from build123d import *

# Parameters (mm, degrees)
SKETCH1_W           = 154
SKETCH1_H           = 104
BOSS_EXTRUDE1_DEPTH = 3
FILLET1_R           = 1
SKETCH2_W           = 149
SKETCH2_H           = 99
SKETCH2_W_2         = 145
SKETCH2_H_2         = 95
EXTRUDE_THIN1_DEPTH = 5
FILLET2_R           = 3
FILLET3_R           = 1
CUT_REVOLVE1_ANGLE  = 90
SKETCH5_W           = 50
SKETCH5_H           = 15
CUT_EXTRUDE1_DEPTH  = 1
FILLET4_R           = 0.5
SKETCH6_R           = 2
CUT_EXTRUDE2_DEPTH  = 5
FILLET5_R           = 0.5


with BuildPart() as part:
    # Sketch1 → Boss-Extrude1 (new body)
    with BuildSketch(Plane(origin=(0, 0, 0), x_dir=(1, 0, 0), z_dir=(0, 1, 0))):
        Rectangle(SKETCH1_W, SKETCH1_H)
    extrude(amount=BOSS_EXTRUDE1_DEPTH)

    # Fillet1
    fillet1_edges = [part.edges().sort_by_distance(p)[0] for p in [
        (-77, 3, 0),
        (0, 3, 52),
        (77, 3, 0),
        (77, 1.5, 52),
        (-77, 1.5, 52),
        (-77, 1.5, -52),
        (77, 1.5, -52),
        (0, 3, -52),
    ]]
    fillet(fillet1_edges, radius=FILLET1_R)

    # Sketch2 → Extrude-Thin1 (add)
    with BuildSketch(Plane.XZ):
        Rectangle(SKETCH2_W, SKETCH2_H)
        Rectangle(SKETCH2_W_2, SKETCH2_H_2, mode=Mode.SUBTRACT)
    extrude(amount=EXTRUDE_THIN1_DEPTH)

    # Fillet2
    fillet2_edges = [part.edges().sort_by_distance(p)[0] for p in [
        (72.5, 0, 0),
        (0, 0, 47.5),
        (-72.5, 0, 0),
        (0, 0, -47.5),
    ]]
    fillet(fillet2_edges, radius=FILLET2_R)

    # Fillet3
    fillet3_edges = [part.edges().sort_by_distance(p)[0] for p in [
        (72.5, -5, 0),
        (0, -5, 47.5),
        (-72.5, -5, 0),
        (0, -5, -47.5),
    ]]
    fillet(fillet3_edges, radius=FILLET3_R)

    # Sketch3 → Cut-Revolve1 (revolve, cut)
    with BuildSketch(Plane.ZY.offset(77)):
        with BuildLine():
            Line((-6.5, 0), (6.5, 0))
            ThreePointArc((6.5, 0), (6.060660172, 1.060660172), (5, 1.5))
            Line((5, 1.5), (-5, 1.5))
            ThreePointArc((-5, 1.5), (-6.060660172, 1.060660172), (-6.5, 0))
        make_face()
    revolve(axis=Axis((-77, 0, -6.5), (0, 0, -1)), revolution_arc=CUT_REVOLVE1_ANGLE, mode=Mode.SUBTRACT)

    # Sketch5 → Cut-Extrude1 (cut)
    with BuildSketch(Plane(origin=(0, 3, 0), x_dir=(1, 0, 0), z_dir=(0, 1, 0))):
        with Locations((0, 33.5)):
            Rectangle(SKETCH5_W, SKETCH5_H)
    extrude(amount=-CUT_EXTRUDE1_DEPTH, mode=Mode.SUBTRACT)

    # Fillet4
    fillet4_edges = [part.edges().sort_by_distance(p)[0] for p in [
        (74.5, -2.5, -49.5),
        (74.5, -2.5, 49.5),
        (-74.5, -2.5, 49.5),
        (-74.5, -2.5, -49.5),
    ]]
    fillet(fillet4_edges, radius=FILLET4_R)

    # Sketch6 → Cut-Extrude2 (cut)
    with BuildSketch(Plane(origin=(0, 2, 0), x_dir=(1, 0, 0), z_dir=(0, 1, 0))):
        with Locations(Location((22, 33.5, 0), (0, 0, 270))):
            Circle(SKETCH6_R)
    extrude(amount=-CUT_EXTRUDE2_DEPTH, mode=Mode.SUBTRACT)

    # Fillet5
    fillet5_edges = [part.edges().sort_by_distance(p)[0] for p in [
        (25, 2, -33.5),
        (0, 2, -26),
        (-25, 2, -33.5),
        (0, 2, -41),
    ]]
    fillet(fillet5_edges, radius=FILLET5_R)


solid = part.part
Here's how the part is built. I have some questions about the finished solid (model axes, mm). A direction names the side the tool comes from. Coordinates: 2 decimals unless noted, no trailing zeros. Order: outer loops, then holes, each group sorted by start corner. A loop starts at its lowest first (then second) coordinate and runs counter-clockwise, first axis right, second up. Notation, with made-up numbers: (-5, 55.25) - (0, 55.25) arc R20 ccw to (0, 82.25) - close; hole circle Ø9 at (60, 38). An arc over 180 degrees is marked (long way). Use CSV: the item, a comma, the result in double quotes. Start each with the question number.
1. For faces 1 (the face through (-1, -2, 49.5)), 2 (the face through (-71.64, -0.9, 0.66)), 3 (the face through (21.234, 1.014, -31.653)), which set-ups out of +Z, -Z, +X, -X, +Y, -Y let a thin tool reach every point of the face, with its end or its side?
2. Please list where these lines run through material, in increasing order: line 1 (X direction, y = 1.45, z = -33.5); line 2 (Z direction, x = 40, y = -4.25); line 3 (Y direction, x = 57, z = 3.5). Write a range as from..to.
3. I'm going to push flat-ended pins straight in: pin 1 (6.5 mm diameter, centred on x = 22, z = -33.5, fed in from -Y); pin 2 (0.5 mm diameter, centred on x = -6.5, y = -3.5, fed in from -Z); pin 3 (1 mm diameter, centred on x = 43, y = -4, fed in from +Z). Where does each tip first touch, or does it pass through?
4. Suppose I cut it at B-B on x = 22. List the corners of the cut face in (y, z) for me.
5. Suppose I cut it at C-C on x = -14. List the corners of the cut face in (y, z) for me.
6. If we mould it in two halves opening along X, with no side actions, what happens to faces 4 (the face through (-1, -2, -49.5)), 5 (the face through (74.5, -2, -1)), 6 (the face through (-74.5, -2, -1)), 7 (the face through (0, 2, -34))? For each: +X half, -X half, draft (parallel to the pull), parting line (faces both ways), or undercut.
7. Suppose I cut it at D-D on z = 35. List the corners of the cut face in (x, y) for me, then the cut area to 3 significant figures.
8. Suppose I cut it at A-A on z = -33.5. List the corners of the cut face in (x, y) for me.
Output:
1,face 1,"+Z, +X, -X, -Y"
1,face 2,"-Y"
1,face 3,"+Y, -Y"
2,line 1,"x = -77..20, 24..77"
2,line 2,"z = -49.5..-47.53, 47.53..49.5"
2,line 3,"y = 0..3"
3,pin 1,"stops at y = 0"
3,pin 2,"stops at z = -49.5"
3,pin 3,"stops at z = 49.5"
4,outline,"(-5, -49.5) - (0, -49.5) - (0, -52) - (2, -52) arc R1 ccw to (3, -51) - (3, -41) - (2.5, -41) arc R0.5 cw to (2, -40.5) - (2, -35.5) - (0, -35.5) - (0, -44.5) arc R3 cw to (-3, -47.5) - (-4, -47.5) arc R1 ccw to (-5, -48.5) - close; (-5, 48.5) arc R1 ccw to (-4, 47.5) - (-3, 47.5) arc R3 cw to (0, 44.5) - (0, -31.5) - (2, -31.5) - (2, -26.5) arc R0.5 cw to (2.5, -26) - (3, -26) - (3, 51) arc R1 ccw to (2, 52) - (0, 52) - (0, 49.5) - (-5, 49.5) - close"
5,outline,"(-5, -49.5) - (0, -49.5) - (0, -52) - (2, -52) arc R1 ccw to (3, -51) - (3, -41) - (2.5, -41) arc R0.5 cw to (2, -40.5) - (2, -26.5) arc R0.5 cw to (2.5, -26) - (3, -26) - (3, 51) arc R1 ccw to (2, 52) - (0, 52) - (0, 49.5) - (-5, 49.5) - (-5, 48.5) arc R1 ccw to (-4, 47.5) - (-3, 47.5) arc R3 cw to (0, 44.5) - (0, -44.5) arc R3 cw to (-3, -47.5) - (-4, -47.5) arc R1 ccw to (-5, -48.5) - close"
6,face 4,"draft"
6,face 5,"+X half"
6,face 6,"-X half"
6,face 7,"undercut"
7,outline,"(-77, 0) - (-74.5, 0) - (-74.5, -5) - (-73.5, -5) arc R1 ccw to (-72.5, -4) - (-72.5, -3) arc R3 cw to (-69.5, 0) - (69.5, 0) arc R3 cw to (72.5, -3) - (72.5, -4) arc R1 ccw to (73.5, -5) - (74.5, -5) - (74.5, 0) - (77, 0) - (77, 2) arc R1 ccw to (76, 3) - (-76, 3) arc R1 ccw to (-77, 2) - close"
7,area,"485 mm2"
8,outline,"(-77, 0) - (-74.5, 0) - (-74.5, -5) - (-73.5, -5) arc R1 ccw to (-72.5, -4) - (-72.5, -3) arc R3 cw to (-69.5, 0) - (20, 0) - (20, 2) - (-24.5, 2) arc R0.5 cw to (-25, 2.5) - (-25, 3) - (-76, 3) arc R1 ccw to (-77, 2) - close; (24, 0) - (69.5, 0) arc R3 cw to (72.5, -3) - (72.5, -4) arc R1 ccw to (73.5, -5) - (74.5, -5) - (74.5, 0) - (77, 0) - (77, 2) arc R1 ccw to (76, 3) - (25, 3) - (25, 2.5) arc R0.5 cw to (24.5, 2) - (24, 2) - close"
